```python
from build123d import *

# Parameters (mm, degrees)
SKETCH3_W           = 17
SKETCH3_H           = 17
BOSS_EXTRUDE1_DEPTH = 0.5
SKETCH4_R           = 5
CUT_EXTRUDE1_DEPTH  = 25.046829313


with BuildPart() as part:
    # Sketch3 → Boss-Extrude1 (new body)
    with BuildSketch(Plane.XY):
        with Locations((8.5, -8.5)):
            Rectangle(SKETCH3_W, SKETCH3_H)
    extrude(amount=BOSS_EXTRUDE1_DEPTH)

    # Sketch4 → Cut-Extrude1 (cut, through all)
    with BuildSketch(Plane.XY.offset(0.5)):
        with Locations((8.5, -8.5)):
            Circle(SKETCH4_R)
        Polygon((17, 0), (14.5, 0), (17, -2.5), align=None)
        Polygon((0, -2.5), (2.5, 0), (0, 0), align=None)
        Polygon((2.5, -17), (0, -14.5), (0, -17), align=None)
        Polygon((17, -17), (17, -14.5), (14.5, -17), align=None)
    extrude(amount=-CUT_EXTRUDE1_DEPTH, mode=Mode.SUBTRACT)


solid = part.part
```
The listing builds one solid part. Answer for the finished solid, in the listing's coordinates (mm). Give positions to 0.01 mm unless a question says otherwise; leave off trailing zeros. Loops run counter-clockwise (first coordinate to the right, second up) from the corner with the lowest first, then second, coordinate; pieces in that order, holes last. Notation, with made-up numbers: M 84,10.25 L 95,10.25 A17 ccw 95,35.25 Z; hole C -36,74.5 d3. An arc over 180 degrees is marked long. One line per item, written item: value.
1. Section A-A on y = -8.5 is taken. Determine the outline of the cut face in (x, z), plus the area to 3 significant figures.
Found:
outline: M 0,0 L 3.5,0 L 3.5,0.5 L 0,0.5 Z; M 13.5,0 L 17,0 L 17,0.5 L 13.5,0.5 Z
area: 3.50 mm^2
2. Section B-B on z = 0.2 is taken. Determine the outline of the cut face in (x, y).
Found:
outline: M 0,-14.5 L 2.5,-17 L 14.5,-17 L 17,-14.5 L 17,-2.5 L 14.5,0 L 2.5,0 L 0,-2.5 Z; hole C 8.5,-8.5 d10
3. This flat-tipped pin is pushed along its axis until it touches: P1, Ø8, axis at x = 9, y = -6, coming from the -Z side. Where does it stop, or does it pass through?
Found:
P1: z = 0
4. Section D-D on y = -1.25 is taken. Determine the outline of the cut face in (x, z), plus the area to 3 significant figures.
Found:
outline: M 1.25,0 L 15.75,0 L 15.75,0.5 L 1.25,0.5 Z
area: 7.25 mm^2
5. For a pull along Y with two mould halves and no side action, classify faces 1 (the face through (13.27, -7, 0.25)), 2 (the face through (1.2, -1.3, 0.3)), 3 (the face through (1.3, -15.8, 0.3)), 4 (the face through (12.2, -12.2, 0.5)) as pulls with the +Y half, pulls with the -Y half, needs draft (parallel to the pull), parting line crosses it, or undercut.
Found:
face 1: undercut
face 2: pulls with the +Y half
face 3: pulls with the -Y half
face 4: needs draft
6. Find the intervals of material crossed by probe 1 along Y at (x, z) = (8.5, 0.2); probe 2 along X at (y, z) = (-6.5, 0.05); probe 3 along Y at (x, z) = (12.25, 0.15), in increasing order.
Found:
probe 1: -17 to -13.5, -3.5 to 0
probe 2: 0 to 3.92, 13.08 to 17
probe 3: -17 to -11.81, -5.19 to 0
7. Section C-C on x = 8.5 is taken. Determine the outline of the cut face in (y, z), plus the area to 3 significant figures.
Found:
outline: M -17,0 L -13.5,0 L -13.5,0.5 L -17,0.5 Z; M -3.5,0 L 0,0 L 0,0.5 L -3.5,0.5 Z
area: 3.50 mm^2
